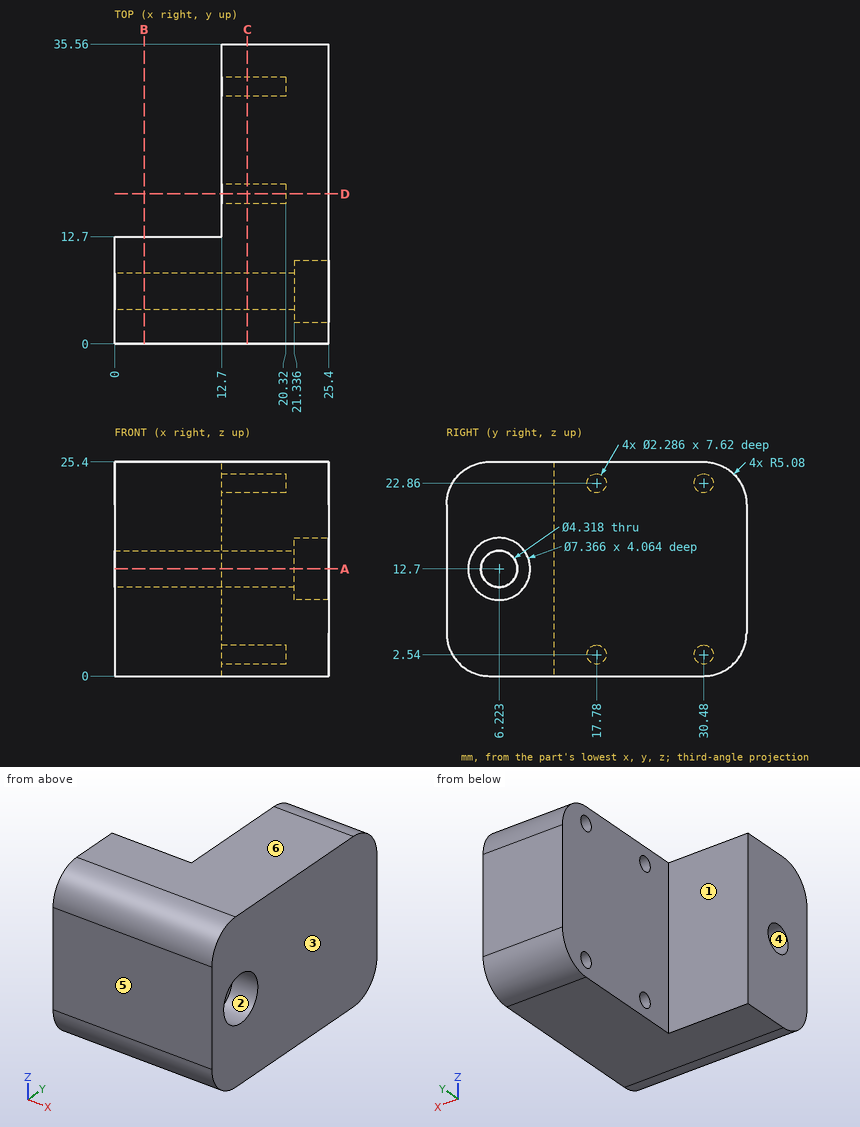
Study the drawing (mm; zero at the part's minimum x, y, z) and answer. A direction names the side the tool comes from. Give positions to 0.01 mm unless a question says otherwise; leave off trailing zeros. Loops run counter-clockwise (first coordinate to the right, second up) from the corner with the lowest first, then second, coordinate; pieces in that order, holes last. Notation, with made-up numbers: M 74,-35 L 122,-35 A10 ccw 122,-27 Z; hole C 32.25,50 d11. An arc over 180 degrees is marked long. One line per item, written item: value.
1. Section D-D on y = 17.78 is taken. Determine the outline of the cut face in (x, z), plus the area to 3 significant figures.
Found:
outline: M 12.7,0 L 25.4,0 L 25.4,25.4 L 12.7,25.4 L 12.7,24 L 20.32,24 L 20.32,21.72 L 12.7,21.72 L 12.7,3.68 L 20.32,3.68 L 20.32,1.4 L 12.7,1.4 Z
area: 288 mm^2
2. For a pull along Z with two mould halves and no side action, classify the marked faces 4, 5 and 6 as pulls with the +Z half, pulls with the -Z half, needs draft (parallel to the pull), parting line crosses it, or undercut.
Found:
face 4: undercut
face 5: needs draft
face 6: pulls with the +Z half
3. Each of these flat-tipped pins is pushed along its axis until it touches: P1, Ø9.5, axis at y = 6.223, z = 12.7, coming from the -X side; P2, Ø11.5, axis at y = 29, z = 8.5, coming from the -X side; P3, Ø10, axis at x = 7, z = 22.5, coming from the +Y side; P4, Ø0.7, axis at y = 30.5, z = 23.5, coming from the -X side. Where does it stop, or does it pass through?
Found:
P1: x = 0
P2: x = 12.7
P3: y = 12.7
P4: x = 20.32
4. Find the intervals of material crossed by probe 1 along Z at (x, y) = (15.5, 17.78); probe 2 along Y at (x, z) = (13, 2); probe 3 along Y at (x, z) = (16.25, 22.86), in increasing order.
Found:
probe 1: 0 to 1.4, 3.68 to 21.72, 24 to 25.4
probe 2: 1.04 to 16.77, 18.79 to 29.47, 31.49 to 34.52
probe 3: 0.68 to 16.64, 18.92 to 29.34, 31.62 to 34.88
5. For the marked faces 1, 2 and 3, determine the directions among +Z, -Z, +X, -X, +Y, -Y from which every point of the face is accessible in a straight line to the end or side of a thin tool.
Found:
face 1: +Z, -Z, -X, +Y
face 2: +X
face 3: +Z, -Z, +X, +Y, -Y
6. Section A-A on z = 12.7 is taken. Determine the outline of the cut face in (x, y).
Found:
outline: M 0,0 L 25.4,0 L 25.4,2.54 L 21.34,2.54 L 21.34,4.06 L 0,4.06 Z; M 0,8.38 L 21.34,8.38 L 21.34,9.91 L 25.4,9.91 L 25.4,35.56 L 12.7,35.56 L 12.7,12.7 L 0,12.7 Z
7. Section B-B on x = 3.5 is taken. Determine the outline of the cut face in (y, z), plus the area to 3 significant figures.
Found:
outline: M 0,5.08 A5.08 ccw 5.08,0 L 12.7,0 L 12.7,25.4 L 5.08,25.4 A5.08 ccw 0,20.32 Z; hole C 6.22,12.7 d4.32
area: 297 mm^2
8. Section C-C on x = 15.75 is taken. Determine the outline of the cut face in (y, z).
Found:
outline: M 0,5.08 A5.08 ccw 5.08,0 L 30.48,0 A5.08 ccw 35.56,5.08 L 35.56,20.32 A5.08 ccw 30.48,25.4 L 5.08,25.4 A5.08 ccw 0,20.32 Z; hole C 6.22,12.7 d4.32; hole C 17.78,2.54 d2.29; hole C 17.78,22.86 d2.29; hole C 30.48,2.54 d2.29; hole C 30.48,22.86 d2.29
